Model file for the job. Use its own axes, mm. A direction names the side the tool comes from. Coordinates: 2 decimals unless noted, no trailing zeros. Write each loop counter-clockwise with the first axis right and the second up, starting at its lowest first coordinate (ties: lowest second). Pieces come first, ordered by that corner, then holes. Notation, with made-up numbers: M 27,79 L 76,79 A6 ccw 76,85 Z; hole C 24.5,57.5 d3. An arc over 180 degrees is marked long. Answer in a Markdown table with one row per item. Add a question column.
Autodesk Fusion 360 part; units mm, degrees
sketch "Sketch1" plane through (0, 0, 0) normal (0, 1, 0) x (1, 0, 0)
  line L0 (-29.9142, 7) -> (-29.9142, 0)
  line L1 (-29.9142, 0) -> (0, 0)
  line L2 (0, 0) -> (0, 7)
  line L3 (-4, 7) -> (-4, 82.0708)
  line L4 (-4, 82.0708) -> (-25.9976, 82.0708)
  line L5 (-25.9976, 82.0708) -> (-25.9976, 7)
  line L6 (0, 7) -> (-4, 7)
  line L7 (-25.9976, 7) -> (-29.9142, 7)
extrude "Extrude1" add sketch "Sketch1" along normal blind 2
fillet "Fillet1" radius 1 2 edges at (-14.9571, 2, 0) (-14.9571, 0, 0)
fillet "Fillet2" radius 1 2 edges at (-14.9988, 2, -82.0708) (-14.9988, 0, -82.0708)
fillet "Fillet3" radius 1 2 edges at (-2, 0, -7) (-2, 2, -7)
fillet "Fillet4" radius 1 2 edges at (-27.9559, 0, -7) (-27.9559, 2, -7)
sketch "Sketch2" plane through (0, 2, 0) normal (0, 1, 0) x (-1, 0, 0)
  line L0 (25.9976, -6) -> (29.9142, -6)
  line L1 (29.9142, -6) -> (29.9142, -1)
  line L2 (29.9142, -1) -> (0, -1)
  line L3 (0, -1) -> (0, -6)
  line L4 (0, -6) -> (4, -6)
  line L5 (4, -6) -> (4, -81.0708)
  line L6 (4, -81.0708) -> (25.9976, -81.0708)
  line L7 (25.9976, -81.0708) -> (25.9976, -6)
  line L8 (13.1427, -55.9691) -> (13.1729, -60.7147)
  line L9 (13.1729, -60.7147) -> (14.0777, -61.0465)
  spline S0 degree 3 poles (14.0777, -61.0464) (14.5804, -61.2274) (15.0429, -61.3782) (15.1033, -61.3782) knots 0 0 0 0 1 1 1 1
  spline S1 degree 3 poles (15.1033, -61.3782) (15.2038, -61.3883) (15.234, -60.4432) (15.2541, -57.1454) knots 0 0 0 0 1 1 1 1
  spline S2 degree 3 poles (15.2541, -57.1454) (15.2842, -53.1238) (15.2943, -52.8925) (15.4652, -52.8624) knots 0 0 0 0 1 1 1 1
  spline S3 degree 3 poles (15.4652, -52.8624) (15.5657, -52.8422) (15.7367, -52.9026) (15.8473, -53.0031) knots 0 0 0 0 1 1 1 1
  spline S4 degree 3 poles (15.8473, -53.0031) (16.0182, -53.164) (16.0383, -53.3248) (16.0383, -55.024) knots 0 0 0 0 1 1 1 1
  line L10 (16.0383, -55.024) -> (16.0383, -56.874)
  line L11 (16.0383, -56.874) -> (16.3902, -57.0248)
  spline S5 degree 3 poles (16.3902, -57.0248) (17.1443, -57.3365) (17.8179, -57.0952) (18.1698, -56.3813) knots 0 0 0 0 1 1 1 1
  spline S6 degree 3 poles (18.1698, -56.3813) (18.3608, -55.9892) (18.401, -55.7479) (18.401, -55.0039) knots 0 0 0 0 1 1 1 1
  spline S7 degree 3 poles (18.401, -55.0039) (18.401, -54.1895) (18.3709, -54.0488) (18.0994, -53.5561) knots 0 0 0 0 1 1 1 1
  spline S8 degree 3 poles (18.0994, -53.5561) (17.8179, -53.0333) (17.3453, -52.611) (16.7119, -52.2792) knots 0 0 0 0 1 1 1 1
  spline S9 degree 3 poles (16.7119, -52.2792) (16.4505, -52.1385) (13.394, -51.2336) (13.203, -51.2336) knots 0 0 0 0 1 1 1 1
  spline S10 degree 3 poles (13.203, -51.2336) (13.1527, -51.2336) (13.1326, -53.3651) (13.1427, -55.9691) knots 0 0 0 0 1 1 1 1
  spline S11 degree 3 poles (10.8604, -57.6079) (8.9602, -58.3117) (8.6284, -58.4625) (8.3569, -58.7642) knots 0 0 0 0 1 1 1 1
  spline S12 degree 3 poles (8.3569, -58.7642) (8.1156, -59.0256) (8.2061, -59.4177) (8.558, -59.6389) knots 0 0 0 0 1 1 1 1
  spline S13 degree 3 poles (8.558, -59.6389) (9.1914, -60.0611) (11.0112, -60.3728) (12.0568, -60.2421) knots 0 0 0 0 1 1 1 1
  line L12 (12.0568, -60.2421) -> (12.6199, -60.1717)
  line L13 (12.6199, -60.1717) -> (12.6199, -59.6188)
  spline S14 degree 3 poles (12.6199, -59.6188) (12.6199, -59.3171) (12.5897, -59.0758) (12.5495, -59.0758) knots 0 0 0 0 1 1 1 1
  spline S15 degree 3 poles (12.5495, -59.0758) (12.5193, -59.0758) (12.1473, -59.1965) (11.7351, -59.3372) knots 0 0 0 0 1 1 1 1
  spline S16 degree 3 poles (11.7351, -59.3372) (11.1821, -59.5283) (10.8906, -59.5785) (10.5889, -59.5283) knots 0 0 0 0 1 1 1 1
  spline S17 degree 3 poles (10.5889, -59.5283) (9.9254, -59.4076) (10.1466, -59.1965) (11.4636, -58.6837) knots 0 0 0 0 1 1 1 1
  line L14 (11.4636, -58.6837) -> (12.6701, -58.2212)
  line L15 (12.6701, -58.2212) -> (12.7003, -57.5878)
  spline S18 degree 3 poles (12.7003, -57.5878) (12.7204, -57.246) (12.6903, -56.9645) (12.65, -56.9745) knots 0 0 0 0 1 1 1 1
  spline S19 degree 3 poles (12.65, -56.9745) (12.6098, -56.9745) (11.8055, -57.2661) (10.8604, -57.6079) knots 0 0 0 0 1 1 1 1
  spline S20 degree 3 poles (16.9934, -57.5778) (16.722, -57.618) (16.2997, -57.7085) (16.0685, -57.7788) knots 0 0 0 0 1 1 1 1
  line L16 (16.0685, -57.7788) -> (15.6361, -57.8995)
  line L17 (15.6361, -57.8995) -> (15.6361, -58.543)
  spline S21 degree 3 poles (15.6361, -58.543) (15.6361, -59.1261) (15.6562, -59.1965) (15.8171, -59.1462) knots 0 0 0 0 1 1 1 1
  spline S22 degree 3 poles (15.8171, -59.1462) (15.9076, -59.1161) (16.4606, -58.925) (17.0437, -58.7239) knots 0 0 0 0 1 1 1 1
  spline S23 degree 3 poles (17.0437, -58.7239) (17.6269, -58.5229) (18.2804, -58.3419) (18.5116, -58.3017) knots 0 0 0 0 1 1 1 1
  spline S24 degree 3 poles (18.5116, -58.3017) (18.9942, -58.2413) (19.4265, -58.4123) (19.2657, -58.6133) knots 0 0 0 0 1 1 1 1
  spline S25 degree 3 poles (19.2657, -58.6133) (19.2054, -58.6837) (18.3709, -59.0256) (17.3956, -59.3775) knots 0 0 0 0 1 1 1 1
  line L18 (17.3956, -59.3775) -> (15.6361, -60.0109)
  line L19 (15.6361, -60.0109) -> (15.6361, -60.6342)
  line L20 (15.6361, -60.6342) -> (15.6361, -61.2576)
  line L21 (15.6361, -61.2576) -> (18.1095, -60.3728)
  spline S26 degree 3 poles (18.1095, -60.3728) (20.6129, -59.4679) (21.1056, -59.2367) (21.2162, -58.8647) knots 0 0 0 0 1 1 1 1
  spline S27 degree 3 poles (21.2162, -58.8647) (21.4977, -58) (19.0043, -57.2359) (16.9934, -57.5778) knots 0 0 0 0 1 1 1 1
extrude "Extrude2" cut sketch "Sketch2" along normal mid plane 1.6 contours L8 L9 S0 S1 S2 S3 S4 L10 L11 S5 S6 S7 S8 S9 S10 | S11 S12 S13 L12 L13 S14 S15 S16 S17 L14 L15 S18 S19 | S20 L16 L17 S21 S22 S23 S24 S25 L18 L19 L20 L21 S26 S27
1) Which spindle directions (+Z, -Z, +X, -X, +Y, -Y) get a long thin tool onto all of the face, cutting with end or side? Do faces 1 (the face through (-15, 2, -42)), 2 (the face through (-4, 1, -44)), 3 (the face through (-19, 1.2, -59)). Say none if no direction does.
2) Slice it at B-B (y = 0.4). Give the cut face in (x, z).
3) Slice it at A-A (z = -49). Give the cut face in (x, y).
4) Flat gauge pins, fed straight in: pin 1 Ø3 at (x, z) = (-3, -62) entering from -Y; pin 2 Ø0.9 at (y, z) = (1.5, -56) entering from -X; pin 3 Ø1 at (y, z) = (0.5, -39) entering from +X. Where does each tip first touch, or does it go through?
5) Two-plate mould, pull along Z, no slides. Class faces 4 (the face through (-15, 1.2, -56)), 5 (the face through (-29.914, 1, -4)): released by +Z, released by -Z, zero draft, split by the parting line, or undercut.
6) Drill centre lines: probe 1 along Z at (x, y) = (-11.25, 1.7); probe 2 along X at (y, z) = (1.3, -42); probe 3 along Z at (x, y) = (-2, 0.95). Where is each one in solid material? Low to high.
Ans:
| question | item | result |
|---|---|---|
| 1 | face 1 | +Z, -Z, +X, -X, +Y |
| 1 | face 2 | -Z, +X, +Y, -Y |
| 1 | face 3 | +Y |
| 2 | outline | M -29.91,-6.8 L -26,-6.8 L -26,-81.87 L -4,-81.87 L -4,-6.8 L 0,-6.8 L 0,-0.2 L -29.91,-0.2 Z |
| 3 | outline | M -26,0 L -4,0 L -4,2 L -26,2 Z |
| 4 | pin 1 | stops at y = 0 |
| 4 | pin 2 | stops at x = -26 |
| 4 | pin 3 | stops at x = -4 |
| 5 | face 4 | undercut |
| 5 | face 5 | zero draft |
| 6 | probe 1 | z = -81.79 to -60.27, -59.49 to -58.77, -57.47 to -0.29 |
| 6 | probe 2 | x = -26 to -4 |
| 6 | probe 3 | z = -7 to 0 |
